CAD build for the part. Positions are in the model's coordinates, mm. A direction names the side the tool comes from. Round coordinates to 2 decimals unless told otherwise and drop trailing zeros. Order: outer loops, then holes, each group sorted by start corner. A loop starts at its lowest first (then second) coordinate and runs counter-clockwise, first axis right, second up. Notation, with made-up numbers: M 84,87 L 95,87 A36 cw 95,125 Z; hole C 63.5,-27 d10. An arc over 180 degrees is marked long. Answer as a JSON object with one key per item and string values. Group by question number.
```python
from build123d import *

# Parameters (mm, degrees)
F0_W   = 1.5
F0_H   = 13
F0_H_2 = 2
F0_W_2 = 0.8


with BuildPart() as f1:
    # F0 (on Front) → F1 (revolve)
    with BuildSketch(Plane.XZ):
        with Locations((19.25, 6.5)):
            Rectangle(F0_W, F0_H)
        with Locations((22.25, 6.5)):
            Rectangle(F0_W, F0_H)
        with Locations((22.25, 14)):
            Rectangle(F0_W, F0_H_2)
        Polygon((20, 15), (20, 13), (21.5, 13), (21.5, 15), (21.15, 15), (20.35, 15), align=None)
        with Locations((19.25, 14)):
            Rectangle(F0_W, F0_H_2)
        with Locations((20.75, 21.5)):
            Rectangle(F0_W_2, F0_H)
    revolve(axis=Axis((0, 0, 7.5), (0, 0, 1)))


solid = f1.part
```
Item 1: Cut at B-B, the plane x = -16. Give the cut face in (y, z), and give its area (3 significant figures).
Item 2: Cut at D-D, the plane z = 25.5. Give the cut face in (x, y), and give its area (3 significant figures).
Item 3: Cut at A-A, the plane y = 0. Give the cut face in (x, z), and give its area (3 significant figures).
Item 4: Cut at C-C, the plane z = 12. Give the cut face in (x, y).
Item 5: 3-axis set-ups, long thin cutter, end or side, ignore diameter. For faces 4 (the face through (-2.799, 21.317, 6.409)), 5 (the face through (-5, -18, 15)), 6 (the face through (-2.994, 22.804, 7.605)): which of +Z, -Z, +X, -X, +Y, -Y reach the whole face in a straight line?
Item 6: Drill centre lines: line 1 (Y direction, x = 0, z = 4.5); line 2 (Y direction, x = 13.5, z = 7.5); line 3 (X direction, y = -10, z = 11.75). Where is each one in solid material? Low to high. Write a range as [from, to].
Item 7: Two-plate mould, pull along Y, no slides. Class faces 1 (the face through (11.1, 17.3, 28)), 2 (the face through (-4.411, -19.866, 21.591)), 3 (the face through (-4.58, -20.65, 21.59)): +Y half, -Y half, draft (parallel to the pull), parting line (faces both ways), or undercut.
Item 8: Flat gauge pins, fed straight in: pin 1 Ø8 at (x, z) = (11.5, 20) entering from -Y; pin 2 Ø4 at (x, z) = (3, 9.5) entering from -Y; pin 3 Ø10 at (x, y) = (-8.5, 8) entering from +Z; pin 4 Ø8 at (y, z) = (-13.5, 17) entering from +X. Where does each tip first touch, or does it go through?
Response values:
{
 "1": {"outline": "M -16.52,0 L -14.36,0 L -14.36,13 L -12,13 L -12,0 L -9.29,0 L -9.29,15 L -12.57,15 L -12.57,28 L -13.83,28 L -13.83,15 L -16.52,15 Z; M 9.29,0 L 12,0 L 12,13 L 14.36,13 L 14.36,0 L 16.52,0 L 16.52,15 L 13.83,15 L 13.83,28 L 12.57,28 L 12.57,15 L 9.29,15 Z", "area": "188 mm^2"},
 "2": {"outline": "C 0,0 d42.3; hole C 0,0 d40.7", "area": "104 mm^2"},
 "3": {"outline": "M -23,0 L -21.5,0 L -21.5,13 L -20,13 L -20,0 L -18.5,0 L -18.5,15 L -20.35,15 L -20.35,28 L -21.15,28 L -21.15,15 L -23,15 Z; M 18.5,0 L 20,0 L 20,13 L 21.5,13 L 21.5,0 L 23,0 L 23,15 L 21.15,15 L 21.15,28 L 20.35,28 L 20.35,15 L 18.5,15 Z", "area": "117 mm^2"},
 "4": {"outline": "C 0,0 d46; C 0,0 d40; hole C 0,0 d43; hole C 0,0 d37"},
 "5": {"face 4": "-Z", "face 5": "+Z", "face 6": "+Z, -Z"},
 "6": {"line 1": "[-23, -21.5], [-20, -18.5], [18.5, 20], [21.5, 23]", "line 2": "[-18.62, -16.73], [-14.76, -12.65], [12.65, 14.76], [16.73, 18.62]", "line 3": "[-20.71, -19.03], [-17.32, -15.56], [15.56, 17.32], [19.03, 20.71]"},
 "7": {"face 1": "draft", "face 2": "undercut", "face 3": "parting line"},
 "8": {"pin 1": "y = -19.78", "pin 2": "y = -22.98", "pin 3": "through", "pin 4": "x = 20.69"}
}
